from build123d import *

# Parameters (mm, degrees)
CORTAR_EXTRUIR1_DEPTH = 345.174069344


with BuildPart() as part:
    # Croquis2 → Revolución1 (revolve)
    with BuildSketch(Plane.XY):
        with BuildLine():
            Line((3.175, 330), (12.7, 330))
            Line((12.7, 330), (12.7, 347.7))
            add(Edge.make_bspline(
                [(12.7, 347.7), (18.502741551, 347.7), (18.502741551, 342.7)],
                knots=[0, 0, 0, 1, 1, 1], degree=2))
            Line((18.502741551, 342.7), (22.5, 342.7))
            Line((22.5, 342.7), (22.5, 347.7))
            add(Edge.make_bspline(
                [(7.5, 362.7), (13.78939178, 362.7), (19.76753999, 357.472351461), (22.5, 349.738947382), (22.5, 347.7)],
                knots=[0, 0, 0, 0, 0.720044841, 1, 1, 1, 1], degree=3))
            Line((7.5, 362.7), (7.5, 350))
            Line((7.5, 350), (0, 350))
            Line((0, 350), (0, 0))
            Line((0, 0), (3.175, 0))
            Line((3.175, 0), (3.175, 330))
        make_face()
    revolve(axis=Axis((0, 0, 0), (0, 1, 0)))

    # Croquis3 → Cortar-Extruir1 (cut, through all)
    with BuildSketch(Plane.XZ.offset(-342.7)):
        with BuildLine():
            ThreePointArc((20.772727273, 8.645449766), (19.5, 0), (20.772727273, -8.645449766))
            ThreePointArc((20.772727273, -8.645449766), (22.5, 0), (20.772727273, 8.645449766))
        make_face()
        with BuildLine():
            ThreePointArc((17.873542761, -13.666984641), (9.75, -16.887495374), (2.899184512, -22.312434407))
            ThreePointArc((2.899184512, -22.312434407), (11.25, -19.485571585), (17.873542761, -13.666984641))
        make_face()
        with BuildLine():
            ThreePointArc((-2.899184512, -22.312434407), (-9.75, -16.887495374), (-17.873542761, -13.666984641))
            ThreePointArc((-17.873542761, -13.666984641), (-11.25, -19.485571585), (-2.899184512, -22.312434407))
        make_face()
        with BuildLine():
            ThreePointArc((-20.772727273, -8.645449766), (-19.5, 0), (-20.772727273, 8.645449766))
            ThreePointArc((-20.772727273, 8.645449766), (-22.5, 0), (-20.772727273, -8.645449766))
        make_face()
        with BuildLine():
            ThreePointArc((-17.873542761, 13.666984641), (-9.75, 16.887495374), (-2.899184512, 22.312434407))
            ThreePointArc((-2.899184512, 22.312434407), (-11.25, 19.485571585), (-17.873542761, 13.666984641))
        make_face()
        with BuildLine():
            ThreePointArc((2.899184512, 22.312434407), (9.75, 16.887495374), (17.873542761, 13.666984641))
            ThreePointArc((17.873542761, 13.666984641), (11.25, 19.485571585), (2.899184512, 22.312434407))
        make_face()
    extrude(amount=-CORTAR_EXTRUIR1_DEPTH, mode=Mode.SUBTRACT)


solid = part.part
Model file for the job. Use its own axes, mm. A direction names the side the tool comes from. Give positions to 0.01 mm unless a question says otherwise; leave off trailing zeros. Loops run counter-clockwise (first coordinate to the right, second up) from the corner with the lowest first, then second, coordinate; pieces in that order, holes last.
Item 1: Mould opens along Z. For faces 1 (the face through (19.5, 347.8, 0.1)), 2 (the face through (3.2, 342.7, -18.4)), 3 (the face through (0, 350, 0)), 4 (the face through (-0.69, 167.31, 3.1)) say: +Z half, -Z half, draft (parallel to the pull), parting line (faces both ways), or undercut.
Check values:
face 1: undercut
face 2: draft
face 3: undercut
face 4: parting line
Item 2: Slice it at A-A (y = 162.5). Write the cut outline in (x, z) (3 decimals), plus the area to 3 significant figures.
Check values:
outline: circle Ø6.35 at (0, 0)
area: 31.7 mm2
Item 3: Drop flat-ended pins along their axis: P1, Ø13.5, axis at x = 0, z = 0, coming from the +Y side; P2, Ø12.5, axis at x = -3, z = -9, coming from the -Y side; P3, Ø10, axis at x = -13.5, z = -17, coming from the +Y side. Give the stop position or say it passes through.
Check values:
P1: stops at y = 350
P2: stops at y = 330
P3: stops at y = 359.2
Item 4: Drill centre lines: line 1 along X through (y, z) = (355, 0); line 2 along Y through (x, z) = (-3.5, 7); line 3 along X through (y, z) = (126, 0) (3 decimals). Where is each one in solid material? Low to high.
Check values:
line 1: x = -19.5 to -7.5, 7.5 to 19.5
line 2: y = 330 to 362.7
line 3: x = -3.175 to 3.175
Item 5: Which spindle directions (+Z, -Z, +X, -X, +Y, -Y) get a long thin tool onto all of the face, cutting with end or side? Do faces 5 (the face through (9.9, 347.8, -16.8)), 6 (the face through (-7.493, 356.261, -0.33)), 7 (the face through (-2.75, 338.97, 12.4)). Say none if no direction does.
Check values:
face 5: -Z, +X, +Y, -Y
face 6: +Y
face 7: -Y
